Input: dimensioned drawing with shaded views. Units: mm. Origin: part minimum x, y, z. A direction names the side the tool comes from. Round coordinates to 2 decimals unless told otherwise and drop trailing zeros. Loops run counter-clockwise (first coordinate to the right, second up) from the corner with the lowest first, then second, coordinate; pieces in that order, holes last. Notation, with made-up numbers: (0, -38.5) - (31, -38.5) arc R23 cw to (31, -30.5) - close; hole circle Ø9 at (-13, 36). An arc over 180 degrees is marked (long way). Answer as a JSON object with one key per item and string values. Group by question number.
Item 1: Section A-A (x = 4). Return the cut outline in (y, z).
Item 2: Section D-D (x = 35). Return the cut outline in (y, z).
Item 3: Line query: line 1 (X direction, y = 30, z = 3.65); line 2 (Y direction, x = 46, z = 3.25); line 3 (Y direction, x = 31.5, z = 3.6). Output: solid intervals per line, ascending.
Item 4: Section C-C (y = 6). Return the cut outline in (x, z).
Item 5: Section B-B (z = 4.05). Return the cut outline in (x, y), plus the area to 3 significant figures.
Item 6: First-contact query: pin 1 (1.5 mm diameter, centred on y = 3.5, z = 2.5, fed in from -X); pin 2 (1.5 mm diameter, centred on y = 2, z = 1.5, fed in from +X); pin 3 (2 mm diameter, centred on x = 31, z = 0.5, fed in from -Y); pin 4 (2.5 mm diameter, centred on x = 57.5, z = 2.5, fed in from +Y). Flat tips, straight axial feed; report the tip coordinate or a pass-through.
Item 7: Draft query along Y for the marked faces 1, 2 and 3. Return one class per face: released by +Y, released by -Y, zero draft, split by the parting line, or undercut.
Item 8: Reachability of the marked faces 4, 5, 6 and 7 from +Z, -Z, +X, -X, +Y, -Y: full face, straight path, thin tool, end or side. Return the list, or none.
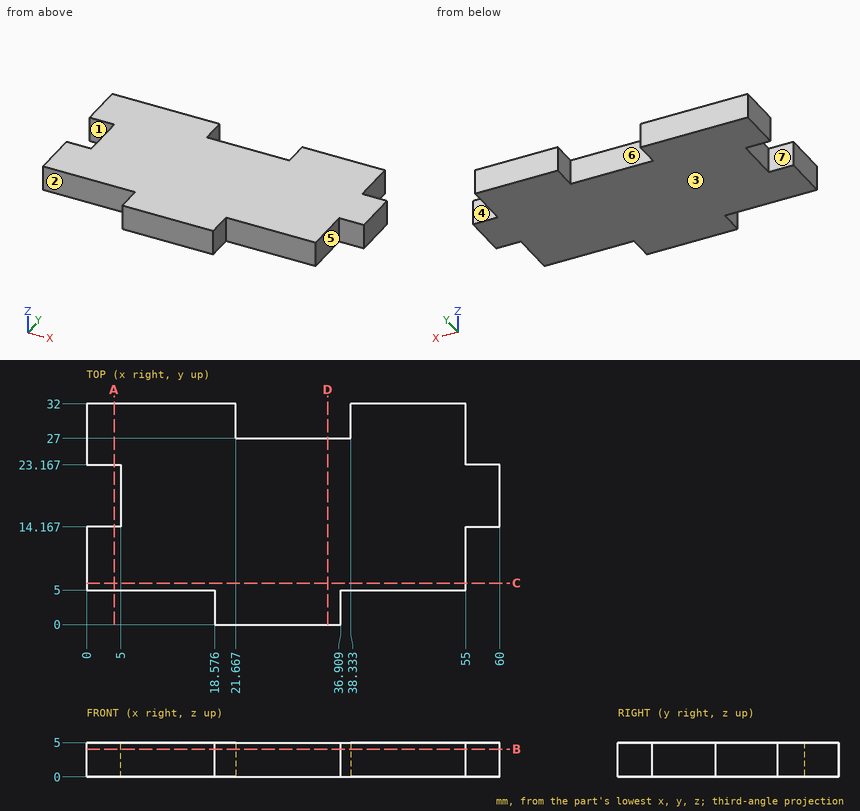
Values:
{
 "1": {"outline": "(5, 0) - (14.17, 0) - (14.17, 5) - (5, 5) - close; (23.17, 0) - (32, 0) - (32, 5) - (23.17, 5) - close"},
 "2": {"outline": "(0, 0) - (27, 0) - (27, 5) - (0, 5) - close"},
 "3": {"line 1": "x = 0 to 21.67, 38.33 to 55", "line 2": "y = 5 to 32", "line 3": "y = 0 to 27"},
 "4": {"outline": "(0, 0) - (55, 0) - (55, 5) - (0, 5) - close"},
 "5": {"outline": "(0, 5) - (18.58, 5) - (18.58, 0) - (36.91, 0) - (36.91, 5) - (55, 5) - (55, 14.17) - (60, 14.17) - (60, 23.17) - (55, 23.17) - (55, 32) - (38.33, 32) - (38.33, 27) - (21.67, 27) - (21.67, 32) - (0, 32) - (0, 23.17) - (5, 23.17) - (5, 14.17) - (0, 14.17) - close", "area": "1,490 mm^2"},
 "6": {"pin 1": "stops at x = 18.58", "pin 2": "stops at x = 36.91", "pin 3": "stops at y = 0", "pin 4": "stops at y = 23.17"},
 "7": {"face 1": "undercut", "face 2": "released by -Y", "face 3": "zero draft"},
 "8": {"face 4": "+Z, -Z, +X, +Y", "face 5": "+Z, -Z, +X, -Y", "face 6": "+Z, -Z, +Y", "face 7": "+Z, -Z, -X"}
}
